```python
from build123d import *

# Parameters (mm, degrees)
F0_W     = 53.975
F0_H     = 104.775
F1_DEPTH = 3.175
F3_W     = 3.175
F3_H     = 101.6
F4_DEPTH = 25.4
F2_R     = 3.175
F5_DEPTH = 25.4


with BuildPart() as f1:
    # F0 (on Top) → F1 (new body)
    with BuildSketch(Plane.XY):
        Rectangle(F0_W, F0_H)
    extrude(amount=F1_DEPTH)

    # F3 (on face) → F4 (join)
    with BuildSketch(Plane.XY.offset(3.175)):
        Polygon((-23.8125, 49.2125), (26.9875, 49.2125), (26.9875, 52.3875), (-26.9875, 52.3875), (-26.9875, 49.2125), align=None)
        with Locations((-25.4, -1.5875)):
            Rectangle(F3_W, F3_H)
    extrude(amount=F4_DEPTH)

    # F2 (on face) → F5 (cut)
    with BuildSketch(Plane.XY.offset(3.175)):
        with Locations((-4.7625, 23.8125)):
            Circle(F2_R)
        with Locations((14.2875, 23.8125)):
            Circle(F2_R)
        with Locations((-4.7625, -1.5875)):
            Circle(F2_R)
        with Locations((14.2875, -1.5875)):
            Circle(F2_R)
        with Locations((-4.7625, -26.9875)):
            Circle(F2_R)
        with Locations((14.2875, -26.9875)):
            Circle(F2_R)
    extrude(amount=-F5_DEPTH, mode=Mode.SUBTRACT)


solid = f1.part
```
Build history of the part. All positions in model axes, mm. A direction names the side the tool comes from. Coordinates: 2 decimals unless noted, no trailing zeros. Order: outer loops, then holes, each group sorted by start corner. A loop starts at its lowest first (then second) coordinate and runs counter-clockwise, first axis right, second up.
Item 1: Drop flat-ended pins along their axis: pin 1 Ø5 at (x, y) = (10.5, -14) entering from +Z (3 decimals); pin 2 Ø5 at (x, y) = (-4.76, -26.99) entering from -Z; pin 3 Ø5 at (y, z) = (-36.5, 7.5) entering from +X; pin 4 Ø1 at (x, z) = (8.5, 8) entering from -Y. Give the stop position or say it passes through.
Filled in:
pin 1: stops at z = 3.175
pin 2: passes through
pin 3: stops at x = -23.81
pin 4: stops at y = 49.21
Item 2: Saw through at B-B on x = 20. List the corners of the cut face in (y, z) (1 decimal).
Filled in:
outline: (-52.4, 0) - (52.4, 0) - (52.4, 28.6) - (49.2, 28.6) - (49.2, 3.2) - (-52.4, 3.2) - close
Item 3: Drill centre lines: L1, parallel to Z at x = 0.5, y = -4 (3 decimals); L2, parallel to Y at x = 7.5, z = 4.5; L3, parallel to X at y = -36, z = 5. Where is each one in solid material? Low to high.
Filled in:
L1: z = 0 to 3.175
L2: y = 49.21 to 52.39
L3: x = -26.99 to -23.81
Item 4: Saw through at A-A on z = 10.75. List the corners of the cut face in (x, y).
Filled in:
outline: (-26.99, -52.39) - (-23.81, -52.39) - (-23.81, 49.21) - (26.99, 49.21) - (26.99, 52.39) - (-26.99, 52.39) - close
Item 5: Mould opens along X. For faces 3 (the cylindrical face through (11.116, -1.448, 1.61)), 4 (the flat face through (26.988, 11, 2)), 5 (the flat face through (-26.988, 1, 14)) say: released by +X, released by -X, zero draft, split by the parting line, or undercut.
Filled in:
face 3: undercut
face 4: released by +X
face 5: released by -X
Item 6: Tool access for faces 1 (the flat face through (-23.812, -2, 16)), 2 (the cylindrical face through (11.77, -28.92, 1.61)): list every direction of +Z, -Z, +X, -X, +Y, -Y with a clear straight run to the whole face (end or side of a thin tool).
Filled in:
face 1: +Z, +X, -Y
face 2: +Z, -Z
